Could you check a few things on this model? Use its own coordinates, in mm. Coordinates: 2 decimals unless noted, no trailing zeros. Loops run counter-clockwise (first coordinate to the right, second up) from the corner with the lowest first, then second, coordinate; pieces in that order, holes last. Notation, with made-up numbers: (38.25, -11) - (94.25, -11) arc R19 ccw to (94.25, 2) - close; hole circle Ø8 at (75.25, 3). An arc over 180 degrees is marked (long way). Put each result on its own line as item: value. Start each with the question number.
Autodesk Inventor part; units mm, degrees
ref_plane "Plano inicial" through (0, 0, 0) normal (0, 0, 1) x (1, 0, 0)
ref_plane "Plano final" through (0, 0, 1019.5555) normal (0, 0, 1) x (1, 0, 0)
ref_plane "Plano de trabalho4" through (-27.5692, 13.7846, 1017.688) normal (0.4452, -0.2226, 0.8673) x (0.8939, 0.0531, -0.4452)
ref_plane "Plano inicial" through (0, 0, 0) normal (0, 0, 1) x (1, 0, 0)
ref_plane "Plano final" through (0, 0, 1019.5555) normal (0, 0, 1) x (1, 0, 0)
sketch "Esboço" plane through (0, 0, 0) normal (0, 0, 1) x (1, 0, 0)
  line L0 (-25.4, -15.875) -> (-25.4, 15.875)
  line L1 (-15.875, 25.4) -> (15.875, 25.4)
  line L2 (25.4, 15.875) -> (25.4, -15.875)
  line L3 (15.875, -25.4) -> (-15.875, -25.4)
  arc A0 (-25.4, -15.875) -> (-15.875, -25.4) centre (-15.875, -15.875) ccw
  arc A1 (-15.875, 25.4) -> (-25.4, 15.875) centre (-15.875, 15.875) ccw
  arc A2 (25.4, 15.875) -> (15.875, 25.4) centre (15.875, 15.875) ccw
  arc A3 (15.875, -25.4) -> (25.4, -15.875) centre (15.875, -15.875) ccw
  arc A4 (-15.875, 20.6375) -> (-20.6375, 15.875) centre (-15.875, 15.875) ccw
  line L4 (-15.875, 20.6375) -> (15.875, 20.6375)
  arc A5 (20.6375, 15.875) -> (15.875, 20.6375) centre (15.875, 15.875) ccw
  line L5 (20.6375, 15.875) -> (20.6375, -15.875)
  arc A6 (15.875, -20.6375) -> (20.6375, -15.875) centre (15.875, -15.875) ccw
  line L6 (15.875, -20.6375) -> (-15.875, -20.6375)
  arc A7 (-20.6375, -15.875) -> (-15.875, -20.6375) centre (-15.875, -15.875) ccw
  line L7 (-20.6375, -15.875) -> (-20.6375, 15.875)
  line L8 (0, 38.3218) -> (0, -38.3218) construction
  line L9 (-38.3218, 0) -> (38.3218, 0) construction
  dimension "d10" = 50.8
  dimension "d11" = 50.8
  dimension "d12" = 4.7625
  dimension "d15" = 25.4
  dimension "d16" = 25.4
  dimension "d17" = 9.525
extrude "Corpo" add sketch "Esboço" along normal up to surface (1019.5555 mm away) from surface at 0
sketch "Sketch3" plane through (0, 0, 0) normal (0, 0, 1) x (1, 0, 0)
  line L0 (0, 0) -> (10, 0)
ref_plane "Work Plane3" through (0, 0, 0) normal (0, -1, 0) x (1, 0, 0)
sketch "Sketch4" plane through (0, 0, 0) normal (0, -1, 0) x (1, 0, 0)
  line L0 (-2, 0) -> (12, 0)
  line L1 (-2, 1019.5555) -> (12, 1019.5555)
  dimension "d19" = 1019.5555
ref_plane "Plano de trabalho4" through (-27.5692, 13.7846, 1017.688) normal (0.4452, -0.2226, 0.8673) x (0.8939, 0.0531, -0.4452)
split "Dividir1" plane through (-27.5692, 13.7846, 1017.688) removes the side toward (0.4452, -0.2226, 0.8673)
equation "\"d10\" = G_H"
equation "\"d11\" = G_W"
equation "\"d12\" = G_T"
equation "\"d15\" = 0.5 * d10"
equation "\"d16\" = 0.5 * d11"
equation "\"d17\" = G_IR"
equation "\"d3\" = G_L"
equation "\"G_W\" = 50.8"
equation "\"G_H\" = 50.8"
equation "\"G_T\" = 4.7625"
equation "\"G_IR\" = 9.525"
equation "\"G_L\" = 1017.40763"
equation "\"G_OFFSET_START\" = 0"
equation "\"G_OFFSET_END\" = 19.55551"
equation "\"d14\" = G_OFFSET_END + B_L"
properties part number "AISC - 2 x 2 x 3/16 - 40,055" material "Aço, suave"
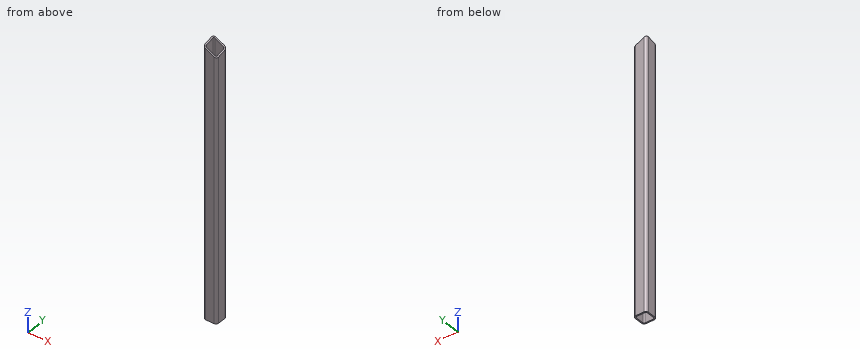
(1) For pin 1 Ø5 at (x, z) = (19, 701.5) entering from +Y, with a flat end and sliding along its axis, tell me the tip position at first contact or that it passes through.
(2) I need wall thicknesses on L1, parallel to X at y = -8, z = 868.5; L2, parallel to Z at x = -23, y = 6. Which ranges of each line are inside material? Lowest first, please. Write a range as [from, to].
(3) I want a section at B-B on y = 1.5. List the corners of the cut face in (x, z) for me.
Answer sheet:
1. pin 1: stops at y = 25.38
2. L1: x = [-25.4, -20.64], [20.64, 25.4]
2. L2: z = [0, 1013.34]
3. outline: (-25.4, 0) - (-20.64, 0) - (-20.64, 1010.98) - (-25.4, 1013.42) - close; (20.64, 0) - (25.4, 0) - (25.4, 987.35) - (20.64, 989.79) - close
